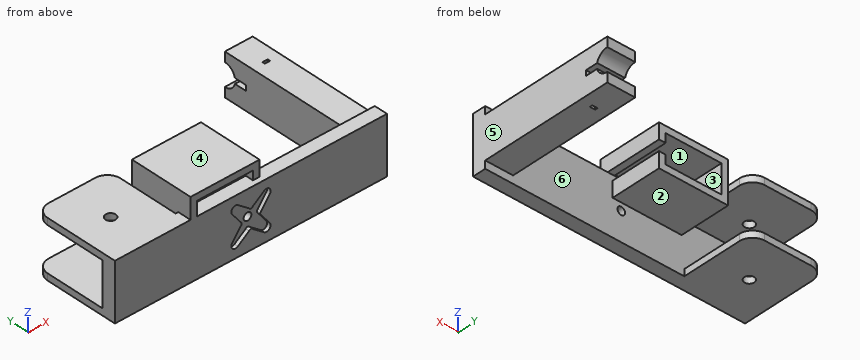
```python
from build123d import *

# Parameters (mm, degrees)
SKETCH1_W           = 205
SKETCH1_H           = 43
BOSS_EXTRUDE1_DEPTH = 10
SKETCH4_W           = 55
SKETCH4_H           = 5
BOSS_EXTRUDE2_DEPTH = 55
SKETCH5_W           = 21
SKETCH5_H           = 31.5
BARREL_STAND_DEPTH  = 100
CUT_EXTRUDE4_DEPTH  = 21
SKETCH7_R           = 3.75
BOLT_HOLE_DEPTH     = 197.370661061
FILLET3_R           = 10
CUT_EXTRUDE9_DEPTH  = 2.8
SKETCH12_R          = 2.9
CUT_EXTRUDE10_DEPTH = 10
SKETCH13_W          = 4
SKETCH13_H          = 2
ZIP_TIE_SLOT_DEPTH  = 196.192210464
BOSS_EXTRUDE3_DEPTH = 38
BOSS_EXTRUDE4_DEPTH = 10


with BuildPart() as part:
    # Sketch1 → Boss-Extrude1 (new body)
    with BuildSketch(Plane(origin=(0, 0, 0), x_dir=(1, 0, 0), z_dir=(0, 1, 0))):
        with Locations((-54.3835126, 22.064427358)):
            Rectangle(SKETCH1_W, SKETCH1_H)
    extrude(amount=BOSS_EXTRUDE1_DEPTH)

    # Sketch4 → Boss-Extrude2 (add)
    with BuildSketch(Plane(origin=(0, 10, 0), x_dir=(1, 0, 0), z_dir=(0, 1, 0))):
        with Locations((-129.3835126, 3.064427358)):
            Rectangle(SKETCH4_W, SKETCH4_H)
    boss_extrude2 = extrude(amount=BOSS_EXTRUDE2_DEPTH)

    # Mirror1: Boss-Extrude2 across plane
    add(boss_extrude2.mirror(Plane.XY.offset(-22.064427358)))

    # Sketch5 → Barrel Stand (add)
    with BuildSketch(Plane(origin=(0, 10, 0), x_dir=(1, 0, 0), z_dir=(0, 1, 0))):
        with Locations((37.6164874, 22.064427358)):
            Rectangle(SKETCH5_W, SKETCH5_H)
    extrude(amount=BARREL_STAND_DEPTH)

    # Sketch6 → Cut-Extrude4 (cut)
    with BuildSketch(Plane(origin=(48.1164874, 0, 10.302060042), x_dir=(0, 0, 1), z_dir=(-1, 0, 0))):
        with BuildLine():
            Line((-34.3664874, 92.5), (-30.3664874, 92.5))
            Line((-30.3664874, 92.5), (-30.3664874, 101.738644179))
            ThreePointArc((-30.3664874, 101.738644179), (-32.3664874, 118.5), (-34.3664874, 101.738644179))
            Line((-34.3664874, 101.738644179), (-34.3664874, 92.5))
        make_face()
    extrude(amount=CUT_EXTRUDE4_DEPTH, mode=Mode.SUBTRACT)

    # Sketch7 → Bolt Hole (cut, through all)
    with BuildSketch(Plane.XY.offset(-0.564427358)):
        with Locations((-130.656969182, 32)):
            Circle(SKETCH7_R)
    extrude(amount=-BOLT_HOLE_DEPTH, mode=Mode.SUBTRACT)

    # Fillet3
    fillet3_edges = [part.edges().sort_by_distance(p)[0] for p in [
        (-156.8835126, 65, -3.064427358),
        (-101.8835126, 65, -3.064427358),
        (-156.8835126, 65, -41.064427358),
        (-101.8835126, 65, -41.064427358),
    ]]
    fillet(fillet3_edges, radius=FILLET3_R)

    # Sketch11 → Cut-Extrude9 (cut)
    # profile 1 of 2: a face of its own
    with BuildSketch(Plane.XZ):
        with BuildLine():
            Line((-40.210281565, -12.15972992), (-46.639894467, -20.689656856))
            ThreePointArc((-46.639894467, -20.689656856), (-47.433748895, -22.064427358), (-46.639894467, -23.43919786))
            Line((-46.639894467, -23.43919786), (-40.210281565, -31.969124796))
            ThreePointArc((-40.210281565, -31.969124796), (-40.489047819, -35.959259074), (-44.479189458, -36.237919954))
            Line((-44.479189458, -36.237919954), (-53.008957608, -29.808073492))
            ThreePointArc((-53.008957608, -29.808073492), (-54.3835126, -29.014191063), (-55.758067592, -29.808073492))
            Line((-55.758067592, -29.808073492), (-64.287835742, -36.237919954))
            ThreePointArc((-64.287835742, -36.237919954), (-68.277977381, -35.959259074), (-68.556743635, -31.969124796))
            Line((-68.556743635, -31.969124796), (-62.127130733, -23.43919786))
            ThreePointArc((-62.127130733, -23.43919786), (-61.333276305, -22.064427358), (-62.127130733, -20.689656856))
            Line((-62.127130733, -20.689656856), (-68.556743635, -12.15972992))
            ThreePointArc((-68.556743635, -12.15972992), (-68.277977381, -8.169595641), (-64.287835742, -7.890934761))
            Line((-64.287835742, -7.890934761), (-55.758067592, -14.320781224))
            ThreePointArc((-55.758067592, -14.320781224), (-54.3835126, -15.114663653), (-53.008957608, -14.320781224))
            Line((-53.008957608, -14.320781224), (-44.479189458, -7.890934761))
            ThreePointArc((-44.479189458, -7.890934761), (-40.489047819, -8.169595641), (-40.210281565, -12.15972992))
        make_face()
        with BuildLine():
            ThreePointArc((-52.857065356, -14.456741186), (-54.3835126, -15.314663653), (-55.909959844, -14.456741186))
            Line((-55.909959844, -14.456741186), (-64.40822508, -8.050642017))
            ThreePointArc((-64.40822508, -8.050642017), (-68.136557893, -8.311018864), (-68.3970332, -12.0393448))
            Line((-68.3970332, -12.0393448), (-61.991158458, -20.537779207))
            ThreePointArc((-61.991158458, -20.537779207), (-61.133276305, -22.064427358), (-61.991158458, -23.591075508))
            Line((-61.991158458, -23.591075508), (-68.3970332, -32.089509915))
            ThreePointArc((-68.3970332, -32.089509915), (-68.136557893, -35.817835851), (-64.40822508, -36.078212699))
            Line((-64.40822508, -36.078212699), (-55.909959844, -29.672113529))
            ThreePointArc((-55.909959844, -29.672113529), (-54.3835126, -28.814191063), (-52.857065356, -29.672113529))
            Line((-52.857065356, -29.672113529), (-44.35880012, -36.078212699))
            ThreePointArc((-44.35880012, -36.078212699), (-40.630467307, -35.817835851), (-40.369992, -32.089509915))
            Line((-40.369992, -32.089509915), (-46.775866742, -23.591075508))
            ThreePointArc((-46.775866742, -23.591075508), (-47.633748895, -22.064427358), (-46.775866742, -20.537779207))
            Line((-46.775866742, -20.537779207), (-40.369992, -12.0393448))
            ThreePointArc((-40.369992, -12.0393448), (-40.630467307, -8.311018864), (-44.35880012, -8.050642017))
            Line((-44.35880012, -8.050642017), (-52.857065356, -14.456741186))
        make_face(mode=Mode.SUBTRACT)
    # profile 2 of 2: a face of its own
    with BuildSketch(Plane.XZ):
        with BuildLine():
            Line((-44.35880012, -8.050642017), (-52.857065356, -14.456741186))
            ThreePointArc((-52.857065356, -14.456741186), (-54.3835126, -15.314663653), (-55.909959844, -14.456741186))
            Line((-55.909959844, -14.456741186), (-64.40822508, -8.050642017))
            ThreePointArc((-64.40822508, -8.050642017), (-68.136557893, -8.311018864), (-68.3970332, -12.0393448))
            Line((-68.3970332, -12.0393448), (-61.991158458, -20.537779207))
            ThreePointArc((-61.991158458, -20.537779207), (-61.133276305, -22.064427358), (-61.991158458, -23.591075508))
            Line((-61.991158458, -23.591075508), (-68.3970332, -32.089509915))
            ThreePointArc((-68.3970332, -32.089509915), (-68.136557893, -35.817835851), (-64.40822508, -36.078212699))
            Line((-64.40822508, -36.078212699), (-55.909959844, -29.672113529))
            ThreePointArc((-55.909959844, -29.672113529), (-54.3835126, -28.814191063), (-52.857065356, -29.672113529))
            Line((-52.857065356, -29.672113529), (-44.35880012, -36.078212699))
            ThreePointArc((-44.35880012, -36.078212699), (-40.630467307, -35.817835851), (-40.369992, -32.089509915))
            Line((-40.369992, -32.089509915), (-46.775866742, -23.591075508))
            ThreePointArc((-46.775866742, -23.591075508), (-47.633748895, -22.064427358), (-46.775866742, -20.537779207))
            Line((-46.775866742, -20.537779207), (-40.369992, -12.0393448))
            ThreePointArc((-40.369992, -12.0393448), (-40.630467307, -8.311018864), (-44.35880012, -8.050642017))
        make_face()
    extrude(amount=-CUT_EXTRUDE9_DEPTH, mode=Mode.SUBTRACT)

    # Sketch12 → Cut-Extrude10 (cut)
    with BuildSketch(Plane(origin=(0, 10, 0), x_dir=(1, 0, 0), z_dir=(0, 1, 0))):
        with Locations(Location((-54.3835126, 22.064427358, 0), (0, 0, 270))):
            Circle(SKETCH12_R)
    extrude(amount=-CUT_EXTRUDE10_DEPTH, mode=Mode.SUBTRACT)

    # Sketch13 → Zip Tie Slot (cut, through all)
    with BuildSketch(Plane.XY.offset(-6.314427358)):
        with Locations((37.6164874, 87.5)):
            Rectangle(SKETCH13_W, SKETCH13_H)
    extrude(amount=-ZIP_TIE_SLOT_DEPTH, mode=Mode.SUBTRACT)

    # Sketch14 → Boss-Extrude3 (add)
    with BuildSketch(Plane(origin=(0, 10, 0), x_dir=(1, 0, 0), z_dir=(0, 1, 0))):
        Polygon((-94.8835126, -10.185572642), (-52.8835126, -10.185572642), (-52.8835126, -3.435572642), (-47.8835126, -3.435572642), (-47.8835126, -15.185572642), (-99.8835126, -15.185572642), (-99.8835126, 16.314427358), (-47.8835126, 16.314427358), (-47.8835126, 4.564427358), (-52.8835126, 4.564427358), (-52.8835126, 11.314427358), (-94.8835126, 11.314427358), align=None)
    extrude(amount=BOSS_EXTRUDE3_DEPTH)

    # Sketch15 → Boss-Extrude4 (add)
    with BuildSketch(Plane.XZ.offset(-10)):
        Polygon((-47.8835126, 15.185572642), (-99.8835126, 15.185572642), (-99.8835126, -0.564427358), (-94.8835126, -0.564427358), (-94.8835126, 10.185572642), (-52.8835126, 10.185572642), (-52.8835126, 3.435572642), (-47.8835126, 3.435572642), align=None)
    extrude(amount=BOSS_EXTRUDE4_DEPTH)


solid = part.part
```
For this review, take the finished solid that the model builds, in its own axes (mm). Face numbers are marked on the shaded views. A direction names the side the tool comes from. Round coordinates to 2 decimals unless told otherwise and drop trailing zeros. Write each loop counter-clockwise with the first axis right and the second up, starting at its lowest first coordinate (ties: lowest second). Pieces come first, ordered by that corner, then holes. Notation, with made-up numbers: (56.25, 64.5) -> (63.25, 64.5) arc R19 cw to (63.25, 94.5) -> close; hole circle Ø6 at (14, -0.5). An arc over 180 degrees is marked (long way). One line per question, with ' | ' between items. Start each with the question number.
(1) Add section D-D, the plane x = -105.5. Write out the cut boundary in (y, z).
(2) Mouldability with a two-part tool opening along Z and no side actions: class the marked faces 4, 5 and 6 as released by +Z, released by -Z, zero draft, split by the parting line, or undercut.
(3) Tool access review of the marked faces 1, 2 and 3: name each direction out of +Z, -Z, +X, -X, +Y, -Y from which nothing blocks a thin tool from reaching the whole face with its end or side.
(4) Insertion check: P1, Ø4, axis at y = 41, z = -41.5, coming from the +X side; P2, Ø5, axis at x = 13.5, z = -34.5, coming from the +Y side; P3, Ø21, axis at x = -77, y = 35.5, coming from the -Z side. Each pin has a flat end and moves straight along its axis. Give the tip position at first contact, or say it passes through.
(5) For line 1 along X through (y, z) = (23, -7); line 2 along Z through (x, y) = (-120.5, 60.5); line 3 along Z through (x, y) = (-65, 12), list the stretches that pass through material, from the lowest coordinate up. Write a range as from..to.
(6) Add section A-A, the plane y = 32. Give the number of separate pieces and of enclosed holes in the cut face, plus the area to 3 significant figures.
(7) Add section C-C, the plane y = 63. Write out the cut boundary in (x, z).
(8) Add section B-B, the plane x = -129.5. Write out the cut boundary in (y, z), plus the area to 3 significant figures.
Answer list:
1) outline: (0, -43.56) -> (62.7, -43.56) -> (62.7, -38.56) -> (10, -38.56) -> (10, -5.56) -> (62.7, -5.56) -> (62.7, -0.56) -> (0, -0.56) -> close
2) face 4: released by +Z | face 5: zero draft | face 6: undercut
3) face 1: +Y, -Y | face 2: -Z, -X, +Y | face 3: +Y
4) P1: x = -101.88 | P2: y = 10 | P3: z = -16.31
5) line 1: -99.88..-94.88, -52.88..-47.88, 27.12..48.12 | line 2: -43.56..-38.56, -5.56..-0.56 | line 3: -16.31..-11.31, 10.19..15.19
6) separate pieces: 6 | enclosed holes: 0 | area: 1,830 mm²
7) outline: (-152.88, -43.56) -> (-105.88, -43.56) -> (-105.88, -38.56) -> (-152.88, -38.56) -> close; (-152.88, -5.56) -> (-105.88, -5.56) -> (-105.88, -0.56) -> (-152.88, -0.56) -> close; (27.12, -37.81) -> (48.12, -37.81) -> (48.12, -6.31) -> (27.12, -6.31) -> close
8) outline: (0, -43.56) -> (28.43, -43.56) -> (28.43, -38.56) -> (10, -38.56) -> (10, -5.56) -> (28.43, -5.56) -> (28.43, -0.56) -> (0, -0.56) -> close; (35.57, -43.56) -> (65, -43.56) -> (65, -38.56) -> (35.57, -38.56) -> close; (35.57, -5.56) -> (65, -5.56) -> (65, -0.56) -> (35.57, -0.56) -> close | area: 909 mm²
